```python
from build123d import *

# Parameters (mm, degrees)
F0_W     = 394
F0_H     = 50
F1_DEPTH = 18
F0_H_2   = 90
F0_H_3   = 110
F0_H_4   = 200
F0_W_2   = 6
F0_H_5   = 314
F0_H_6   = 18
F0_H_7   = 6
F2_DEPTH = 9


with BuildPart() as f1:
    # F0 (on Right) → F1 (new body)
    with BuildSketch(Plane.YZ):
        with Locations((203, 775)):
            Rectangle(F0_W, F0_H)
    extrude(amount=F1_DEPTH)



with BuildPart() as f1b:
    # F0 (on Right) → F1, piece 2 (new body)
    with BuildSketch(Plane.YZ):
        with Locations((203, 699)):
            Rectangle(F0_W, F0_H_2)
    extrude(amount=F1_DEPTH)


with BuildPart() as f1c:
    # F0 (on Right) → F1, piece 3 (new body)
    with BuildSketch(Plane.YZ):
        with Locations((203, 593)):
            Rectangle(F0_W, F0_H_3)
    extrude(amount=F1_DEPTH)


with BuildPart() as f1d:
    # F0 (on Right) → F1, piece 4 (new body)
    with BuildSketch(Plane.YZ):
        with Locations((203, 432)):
            Rectangle(F0_W, F0_H_4)
    extrude(amount=F1_DEPTH)


with BuildPart() as f1e:
    # F0 (on Right) → F1, piece 5 (new body)
    with BuildSketch(Plane.YZ):
        Polygon((6, 314), (6, 0), (394, 0), (400, 0), (400, 314), align=None)
    extrude(amount=F1_DEPTH)


with BuildPart() as f1_1:
    add(f1.part)

    add(f1b.part)  # F2 merges F1b

    add(f1c.part)  # F2 merges F1c

    add(f1d.part)  # F2 merges F1d

    add(f1e.part)  # F2 merges F1e
    # F0 (on Right) → F2 (join)
    with BuildSketch(Plane.YZ):
        with Locations((3, 157)):
            Rectangle(F0_W_2, F0_H_5)
        with Locations((3, 323)):
            Rectangle(F0_W_2, F0_H_6)
        with Locations((203, 323)):
            Rectangle(F0_W, F0_H_6)
        with Locations((3, 432)):
            Rectangle(F0_W_2, F0_H_4)
        with Locations((203, 535)):
            Rectangle(F0_W, F0_H_7)
        with Locations((203, 651)):
            Rectangle(F0_W, F0_H_7)
        with Locations((3, 593)):
            Rectangle(F0_W_2, F0_H_3)
        with Locations((3, 651)):
            Rectangle(F0_W_2, F0_H_7)
        with Locations((3, 775)):
            Rectangle(F0_W_2, F0_H)
        with Locations((3, 747)):
            Rectangle(F0_W_2, F0_H_7)
        with Locations((3, 699)):
            Rectangle(F0_W_2, F0_H_2)
        with Locations((203, 747)):
            Rectangle(F0_W, F0_H_7)
        with Locations((3, 535)):
            Rectangle(F0_W_2, F0_H_7)
    extrude(amount=F2_DEPTH)


solid = f1_1.part
```
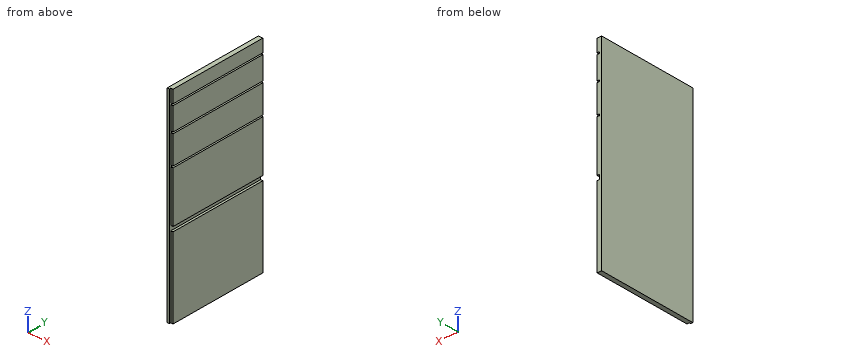
Could you check a few things on this model? Use its own coordinates, in mm. Round coordinates to 2 decimals unless told otherwise and drop trailing zeros. Write each loop counter-clockwise with the first axis right and the second up, starting at its lowest first coordinate (ties: lowest second). Pieces come first, ordered by that corner, then holes.
(1) For pin 1 (4.5 mm diameter, centred on x = 15, z = 577.5, fed in from -Y), with a flat end and sliding along its axis, tell me the tip position at first contact or that it passes through.
Findings below:
pin 1: stops at y = 6
(2) Suppose I cut it at B-B on y = 165.5. Write out the boundary of the cut face in (x, z), and give its area (3 significant figures).
Findings below:
outline: (0, 0) - (18, 0) - (18, 314) - (9, 314) - (9, 332) - (18, 332) - (18, 532) - (9, 532) - (9, 538) - (18, 538) - (18, 648) - (9, 648) - (9, 654) - (18, 654) - (18, 744) - (9, 744) - (9, 750) - (18, 750) - (18, 800) - (0, 800) - close
area: 14,100 mm2
(3) Suppose I cut it at A-A on x = 14.5. Write out the boundary of the cut face in (y, z).
Findings below:
outline: (6, 0) - (400, 0) - (400, 314) - (6, 314) - close; (6, 332) - (400, 332) - (400, 532) - (6, 532) - close; (6, 538) - (400, 538) - (400, 648) - (6, 648) - close; (6, 654) - (400, 654) - (400, 744) - (6, 744) - close; (6, 750) - (400, 750) - (400, 800) - (6, 800) - close
(4) If I drill on probe 1 along Z at (x, y) = (10.75, 92.5); probe 2 along Y at (x, z) = (15.75, 363); probe 3 along X at (y, z) = (309, 748), over which ranges is the centre line in solid material (lowest first)?
Findings below:
probe 1: z = 0 to 314, 332 to 532, 538 to 648, 654 to 744, 750 to 800
probe 2: y = 6 to 400
probe 3: x = 0 to 9
